Check sheet for the modelled part. Datum: model origin and axes. Units: mm. Face numbers are marked on the shaded views. A direction names the side the tool comes from. Round coordinates to 2 decimals unless told otherwise and drop trailing zeros. Loops run counter-clockwise (first coordinate to the right, second up) from the corner with the lowest first, then second, coordinate; pieces in that order, holes last. Notation, with made-up numbers: (13.5, 61.25) - (45.5, 61.25) arc R22 cw to (45.5, 95.25) - close; hole circle Ø6 at (38, 61.5). An arc over 180 degrees is marked (long way). Answer in a Markdown table with one row per item. Add a question column.
(1) Cross-section at B-B on x = 0. Enter the section's corners in (y, z), then the cut area to 4 significant figures.
(2) Gauge pin test, flat ends, axial feed: pin 1 (4 mm diameter, centred on x = 1, z = -9, fed in from +Y); pin 2 (1.1 mm diameter, centred on x = 0, y = 10, fed in from +Z); pin 3 (2.5 mm diameter, centred on x = 0, z = -9, fed in from -Y); pin 4 (3 mm diameter, centred on x = 0.5, z = 1.5, fed in from -Y). Record the tip position at first contact, or that the pin passes through.
(3) Access from +Z, -Z, +X, -X, +Y, -Y to the whole of each face (thin tool, end or side, straight path). Record for the marked faces 4, 5 and 6.
(4) Cross-section at D-D on z = -6.5. Enter the section's corners in (x, y).
(5) Mould release check, pull along Z, two halves, no side actions. Record for the marked faces 1, 2 and 3: +Z half, -Z half, draft (parallel to the pull), parting line (faces both ways), or undercut.
(6) Thickness scan on line 1 along X through (y, z) = (2.5, -9); line 2 along Z through (x, y) = (0.5, 7); line 3 along Y through (x, z) = (4.75, 11). Record the ranges inside material, lowest first.
(7) Cross-section at A-A on y = 5. Enter the section's corners in (x, z), then the cut area to 3 significant figures.
from build123d import *

# Parameters (mm, degrees)
MAIN_DEPTH                      = 12
SKETCH2_R                       = 1.5
HOLEMAKERBEAMFIX_DEPTH          = 17.710774967
SKETCH3_W                       = 10
SKETCH3_H                       = 13.5
MAINCONNECTORHOLE_DEPTH         = 7.3
SKETCH4_W                       = 5
SKETCH4_H                       = 24
CONNECTORSUPPORTEXTENSION_DEPTH = 3.2
SKETCH5_W                       = 1.8
SKETCH5_H                       = 8.5
CONNECTORRAILHOLE_DEPTH         = 1.5
SKETCH6_W                       = 2.9
SKETCH6_H                       = 7
CUT_EXTRUDE4_DEPTH              = 1
FILLET3_R                       = 5


with BuildPart() as part:
    # Sketch1 → Main (new, symmetric)
    with BuildSketch(Plane.XY):
        Polygon((-5, 8.5), (-5, 0), (5, 0), (5, 8.5), (1.45, 8.5), (1.45, 10.5), (-1.45, 10.5), (-1.45, 8.5), align=None)
    extrude(amount=MAIN_DEPTH, both=True)

    # Sketch2 → HoleMakerBeamFix (cut, through all)
    with BuildSketch(Plane(origin=(0, 10.5, 0), x_dir=(1, 0, 0), z_dir=(0, 1, 0))):
        with Locations(Location((0, -9, 0), (0, 0, 270))):
            Circle(SKETCH2_R)
        with Locations(Location((0, 9, 0), (0, 0, 270))):
            Circle(SKETCH2_R)
    extrude(amount=-HOLEMAKERBEAMFIX_DEPTH, mode=Mode.SUBTRACT)

    # Sketch3 → MainConnectorHole (cut)
    with BuildSketch(Plane(origin=(0, 0, 0), x_dir=(-1, 0, 0), z_dir=(0, -1, 0))):
        Rectangle(SKETCH3_W, SKETCH3_H)
    extrude(amount=-MAINCONNECTORHOLE_DEPTH, mode=Mode.SUBTRACT)

    # Sketch4 → ConnectorSupportExtension (add)
    with BuildSketch(Plane(origin=(0, 7.3, 0), x_dir=(-1, 0, 0), z_dir=(0, -1, 0))):
        with Locations((7.5, 0)):
            Rectangle(SKETCH4_W, SKETCH4_H)
    extrude(amount=-CONNECTORSUPPORTEXTENSION_DEPTH)

    # Sketch5 → ConnectorRailHole (cut)
    with BuildSketch(Plane(origin=(0, 7.3, 0), x_dir=(-1, 0, 0), z_dir=(0, -1, 0))):
        with Locations((7.9, 0)):
            Rectangle(SKETCH5_W, SKETCH5_H)
    extrude(amount=-CONNECTORRAILHOLE_DEPTH, mode=Mode.SUBTRACT)

    # Sketch6 → Cut-Extrude4 (cut)
    with BuildSketch(Plane(origin=(0, 10.5, 0), x_dir=(1, 0, 0), z_dir=(0, 1, 0))):
        with Locations((0, 8.5)):
            Rectangle(SKETCH6_W, SKETCH6_H)
        with Locations((0, -8.5)):
            Rectangle(SKETCH6_W, SKETCH6_H)
    extrude(amount=-CUT_EXTRUDE4_DEPTH, mode=Mode.SUBTRACT)

    # Fillet3
    fillet3_edges = [part.edges().sort_by_distance(p)[0] for p in [
        (-5, 7.3, -9.375),
        (-5, 7.3, 9.375),
    ]]
    fillet(fillet3_edges, radius=FILLET3_R - 0.0001)  # a hair under: the kernel refuses the full size


solid = part.part
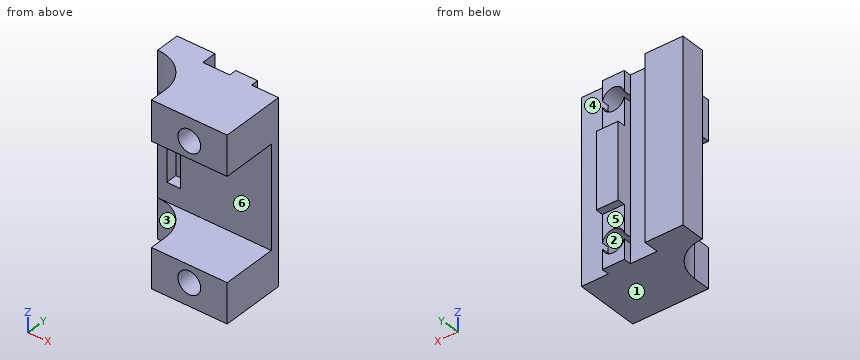
Answers:
| question | item | result |
|---|---|---|
| 1 | outline | (0, -12) - (9.5, -12) - (9.5, -10.5) - (0, -10.5) - close; (0, -7.5) - (9.5, -7.5) - (9.5, -5) - (10.5, -5) - (10.5, 5) - (9.5, 5) - (9.5, 7.5) - (0, 7.5) - (0, 6.75) - (7.3, 6.75) - (7.3, -6.75) - (0, -6.75) - close; (0, 10.5) - (9.5, 10.5) - (9.5, 12) - (0, 12) - close |
| 1 | area | 82.45 mm^2 |
| 2 | pin 1 | stops at y = 9.5 |
| 2 | pin 2 | stops at z = 12 |
| 2 | pin 3 | passes through |
| 2 | pin 4 | stops at y = 7.3 |
| 3 | face 4 | +Z, -Z, +X, +Y |
| 3 | face 5 | -Z, +X, +Y |
| 3 | face 6 | +X, -X, -Y |
| 4 | outline | (-10, 7.3) - (5, 7.3) - (5, 8.5) - (1.45, 8.5) - (1.45, 9.5) - (-1.45, 9.5) - (-1.45, 8.5) - (-5, 8.5) - (-5, 10.5) - (-10, 10.5) - close |
| 5 | face 1 | -Z half |
| 5 | face 2 | undercut |
| 5 | face 3 | draft |
| 6 | line 1 | x = -5 to -1.5, 1.5 to 5 |
| 6 | line 2 | z = -12 to -10.41, -7.59 to -6.75, 6.75 to 7.59, 10.41 to 12 |
| 6 | line 3 | y = 0 to 8.5 |
| 7 | outline | (-5.79, -12) - (5, -12) - (5, -6.75) - (-5.79, -6.75) - close; (-5.79, 6.75) - (5, 6.75) - (5, 12) - (-5.79, 12) - close; hole circle Ø3 at (0, -9); hole circle Ø3 at (0, 9) |
| 7 | area | 99.2 mm^2 |
